from build123d import *

# Parameters (mm, degrees)
F1_DEPTH = 2762.25
F2_W     = 152.146
F2_H     = 254.254
F3_DEPTH = 15.875
F4_W     = 152.146
F4_H     = 254.254
F5_DEPTH = 15.875
F7_DEPTH = 3.175
F8_R     = 9.525
F9_DEPTH = 2794


with BuildPart() as f1:
    # F0 (on Front) → F1 (new body)
    with BuildSketch(Plane.XZ):
        with BuildLine():
            Line((76.073, 76.073), (-76.073, 76.073))
            Line((-76.073, 76.073), (-76.073, 69.469))
            Line((-76.073, 69.469), (-9.271, 69.469))
            ThreePointArc((-9.271, 69.469), (-4.7808719395, 67.6091280605), (-2.921, 63.119))
            Line((-2.921, 63.119), (-2.921, -63.119))
            ThreePointArc((-2.921, -63.119), (-4.7808719395, -67.6091280605), (-9.271, -69.469))
            Line((-9.271, -69.469), (-76.073, -69.469))
            Line((-76.073, -69.469), (-76.073, -76.073))
            Line((-76.073, -76.073), (76.073, -76.073))
            Line((76.073, -76.073), (76.073, -69.469))
            Line((76.073, -69.469), (9.271, -69.469))
            ThreePointArc((9.271, -69.469), (4.7808719395, -67.6091280605), (2.921, -63.119))
            Line((2.921, -63.119), (2.921, 63.119))
            ThreePointArc((2.921, 63.119), (4.7808719395, 67.6091280605), (9.271, 69.469))
            Line((9.271, 69.469), (76.073, 69.469))
            Line((76.073, 69.469), (76.073, 76.073))
        make_face()
    extrude(amount=F1_DEPTH)

    # F2 (on face) → F3 (join)
    with BuildSketch(Plane.XZ.offset(2762.25)):
        with BuildLine():
            Line((9.271, -69.469), (76.073, -69.469))
            Line((76.073, -69.469), (76.073, 69.469))
            Line((76.073, 69.469), (9.271, 69.469))
            ThreePointArc((9.271, 69.469), (4.7808719395, 67.6091280605), (2.921, 63.119))
            Line((2.921, 63.119), (2.921, -63.119))
            ThreePointArc((2.921, -63.119), (4.7808719395, -67.6091280605), (9.271, -69.469))
        make_face()
        with BuildLine():
            Line((-76.073, 69.469), (-76.073, -69.469))
            Line((-76.073, -69.469), (-9.271, -69.469))
            ThreePointArc((-9.271, -69.469), (-4.7808719395, -67.6091280605), (-2.921, -63.119))
            Line((-2.921, -63.119), (-2.921, 63.119))
            ThreePointArc((-2.921, 63.119), (-4.7808719395, 67.6091280605), (-9.271, 69.469))
            Line((-9.271, 69.469), (-76.073, 69.469))
        make_face()
        with Locations((0, 203.2)):
            Rectangle(F2_W, F2_H)
        with BuildLine():
            Line((-76.073, -69.469), (-76.073, -76.073))
            Line((-76.073, -76.073), (76.073, -76.073))
            Line((76.073, -76.073), (76.073, -69.469))
            Line((76.073, -69.469), (9.271, -69.469))
            ThreePointArc((9.271, -69.469), (4.7808719395, -67.6091280605), (2.921, -63.119))
            Line((2.921, -63.119), (2.921, 63.119))
            ThreePointArc((2.921, 63.119), (4.7808719395, 67.6091280605), (9.271, 69.469))
            Line((9.271, 69.469), (76.073, 69.469))
            Line((76.073, 69.469), (76.073, 76.073))
            Line((76.073, 76.073), (-76.073, 76.073))
            Line((-76.073, 76.073), (-76.073, 69.469))
            Line((-76.073, 69.469), (-9.271, 69.469))
            ThreePointArc((-9.271, 69.469), (-4.7808719395, 67.6091280605), (-2.921, 63.119))
            Line((-2.921, 63.119), (-2.921, -63.119))
            ThreePointArc((-2.921, -63.119), (-4.7808719395, -67.6091280605), (-9.271, -69.469))
            Line((-9.271, -69.469), (-76.073, -69.469))
        make_face()
    extrude(amount=F3_DEPTH)

    # F4 (on face) → F5 (join)
    with BuildSketch(Plane(origin=(0, 0, 0), x_dir=(-1, 0, 0), z_dir=(0, 1, 0))):
        with Locations((0, 203.2)):
            Rectangle(F4_W, F4_H)
        with BuildLine():
            Line((-76.073, -76.073), (76.073, -76.073))
            Line((76.073, -76.073), (76.073, -69.469))
            Line((76.073, -69.469), (9.271, -69.469))
            ThreePointArc((9.271, -69.469), (4.7808719395, -67.6091280605), (2.921, -63.119))
            Line((2.921, -63.119), (2.921, 63.119))
            ThreePointArc((2.921, 63.119), (4.7808719395, 67.6091280605), (9.271, 69.469))
            Line((9.271, 69.469), (76.073, 69.469))
            Line((76.073, 69.469), (76.073, 76.073))
            Line((76.073, 76.073), (-76.073, 76.073))
            Line((-76.073, 76.073), (-76.073, 69.469))
            Line((-76.073, 69.469), (-9.271, 69.469))
            ThreePointArc((-9.271, 69.469), (-4.7808719395, 67.6091280605), (-2.921, 63.119))
            Line((-2.921, 63.119), (-2.921, -63.119))
            ThreePointArc((-2.921, -63.119), (-4.7808719395, -67.6091280605), (-9.271, -69.469))
            Line((-9.271, -69.469), (-76.073, -69.469))
            Line((-76.073, -69.469), (-76.073, -76.073))
        make_face()
        with BuildLine():
            Line((9.271, -69.469), (76.073, -69.469))
            Line((76.073, -69.469), (76.073, 69.469))
            Line((76.073, 69.469), (9.271, 69.469))
            ThreePointArc((9.271, 69.469), (4.7808719395, 67.6091280605), (2.921, 63.119))
            Line((2.921, 63.119), (2.921, -63.119))
            ThreePointArc((2.921, -63.119), (4.7808719395, -67.6091280605), (9.271, -69.469))
        make_face()
        with BuildLine():
            Line((-76.073, 69.469), (-76.073, -69.469))
            Line((-76.073, -69.469), (-9.271, -69.469))
            ThreePointArc((-9.271, -69.469), (-4.7808719395, -67.6091280605), (-2.921, -63.119))
            Line((-2.921, -63.119), (-2.921, 63.119))
            ThreePointArc((-2.921, 63.119), (-4.7808719395, 67.6091280605), (-9.271, 69.469))
            Line((-9.271, 69.469), (-76.073, 69.469))
        make_face()
    extrude(amount=F5_DEPTH)

    # F6 (on Right) → F7 (join, symmetric)
    with BuildSketch(Plane.YZ):
        Polygon((0, 76.073), (0, 330.073), (-254, 76.073), align=None)
        Polygon((-2762.25, 330.073), (-2762.25, 76.073), (-2508.25, 76.073), align=None)
    extrude(amount=F7_DEPTH, both=True)

    # F8 (on face) → F9 (cut)
    with BuildSketch(Plane(origin=(0, 15.875, 0), x_dir=(-1, 0, 0), z_dir=(0, 1, 0))):
        with Locations((-37.973, 276.352)):
            Circle(F8_R)
        with Locations((37.973, 127.127)):
            Circle(F8_R)
        with Locations((-37.973, 127.127)):
            Circle(F8_R)
        with Locations((-37.973, -22.098)):
            Circle(F8_R)
        with Locations((37.973, -22.098)):
            Circle(F8_R)
        with Locations((37.973, 276.352)):
            Circle(F8_R)
    extrude(amount=-F9_DEPTH, mode=Mode.SUBTRACT)


solid = f1.part
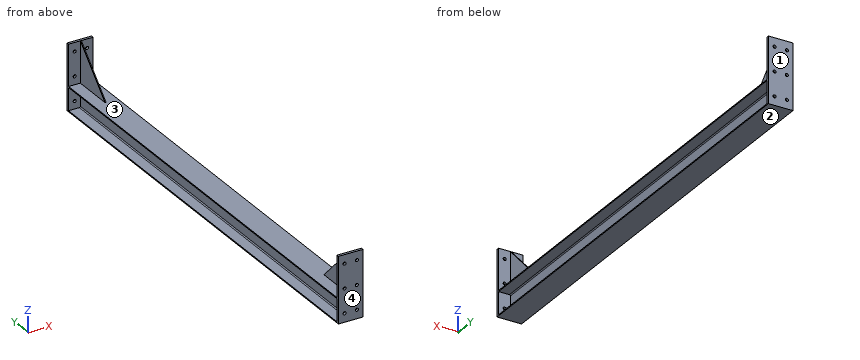
Build history of the part. All positions in model axes, mm. Face numbers are marked on the shaded views. Round coordinates to 2 decimals unless told otherwise and drop trailing zeros. Write each loop counter-clockwise with the first axis right and the second up, starting at its lowest first coordinate (ties: lowest second). Pieces come first, ordered by that corner, then holes. Notation, with made-up numbers: (30.25, 67) -> (71.25, 67) arc R24 cw to (71.25, 88) -> close; hole circle Ø8 at (43.5, 2.25). An arc over 180 degrees is marked (long way). Use one line per item in the form item = value.
Q1. Band-saw the part on C-C, the plane z = 18. Write the cut outline in (x, y) (3 decimals).
Conclusion:
outline = (-76.073, -2778.125) -> (76.073, -2778.125) -> (76.073, -2762.25) -> (2.921, -2762.25) -> (2.921, 0) -> (76.073, 0) -> (76.073, 15.875) -> (-76.073, 15.875) -> (-76.073, 0) -> (-2.921, 0) -> (-2.921, -2762.25) -> (-76.073, -2762.25) -> close
Q2. Band-saw the part on A-A, the plane z = 160. Write the cut outline in (x, y) (3 decimals), then the cut area to 3 significant figures.
Conclusion:
outline = (-76.073, -2778.125) -> (76.073, -2778.125) -> (76.073, -2762.25) -> (3.175, -2762.25) -> (3.175, -2592.177) -> (-3.175, -2592.177) -> (-3.175, -2762.25) -> (-76.073, -2762.25) -> close; (-76.073, 0) -> (-3.175, 0) -> (-3.175, -170.073) -> (3.175, -170.073) -> (3.175, 0) -> (76.073, 0) -> (76.073, 15.875) -> (-76.073, 15.875) -> close
area = 6,990 mm²
Q3. Drill centre lines: L1, parallel to Y at x = 31.5, z = 314 (3 decimals); L2, parallel to Z at x = 12, y = -1988.5; L3, parallel to X at y = -825.5, z = 54. Where is each one in solid material? Low to high.
Conclusion:
L1 = -2778.125 to -2762.25, 0 to 15.875
L2 = -76.07 to -69.47, 69.47 to 76.07
L3 = -2.92 to 2.92
Q4. Drop flat-ended pins along their axis: P1, Ø17, axis at x = -37.973, z = 276.352, coming from the +Y side; P2, Ø10, axis at y = -1154, z = -17, coming from the -X side. Give the stop position or say it passes through.
Conclusion:
P1 = through
P2 = -2.92
Q5. Band-saw the part on B-B, the plane y = -1953.5. Write the cut outline in (x, z).
Conclusion:
outline = (-76.07, -76.07) -> (76.07, -76.07) -> (76.07, -69.47) -> (9.27, -69.47) arc R6.35 cw to (2.92, -63.12) -> (2.92, 63.12) arc R6.35 cw to (9.27, 69.47) -> (76.07, 69.47) -> (76.07, 76.07) -> (-76.07, 76.07) -> (-76.07, 69.47) -> (-9.27, 69.47) arc R6.35 cw to (-2.92, 63.12) -> (-2.92, -63.12) arc R6.35 cw to (-9.27, -69.47) -> (-76.07, -69.47) -> close
Q6. Band-saw the part on D-D, the plane y = -229. Write the cut outline in (x, z) (3 decimals).
Conclusion:
outline = (-76.073, -76.073) -> (76.073, -76.073) -> (76.073, -69.469) -> (9.271, -69.469) arc R6.35 cw to (2.921, -63.119) -> (2.921, 63.119) arc R6.35 cw to (9.271, 69.469) -> (76.073, 69.469) -> (76.073, 76.073) -> (3.175, 76.073) -> (3.175, 101.073) -> (-3.175, 101.073) -> (-3.175, 76.073) -> (-76.073, 76.073) -> (-76.073, 69.469) -> (-9.271, 69.469) arc R6.35 cw to (-2.921, 63.119) -> (-2.921, -63.119) arc R6.35 cw to (-9.271, -69.469) -> (-76.073, -69.469) -> close
Q7. Two-plate mould, pull along Y, no slides. Class the marked faces 1, 2, 3 and 4: released by +Y, released by -Y, zero draft, split by the parting line, or undercut.
Conclusion:
face_1 = released by +Y
face_2 = zero draft
face_3 = undercut
face_4 = released by -Y
